```python
from build123d import *

# Parameters (mm, degrees)
BOSS_EXTRUDE1_DEPTH   = 8
CUT_EXTRUDE2_DEPTH    = 27.019223663
M3X0_5_TAPPED_HOLE1_D = 2.5
SKETCH7_W             = 20.825163494
SKETCH7_H             = 21.535112249
CUT_EXTRUDE3_DEPTH    = 8


with BuildPart() as part:
    # Sketch1 → Boss-Extrude1 (new body)
    with BuildSketch(Plane(origin=(0, 0, 0), x_dir=(0, 0, -1), z_dir=(1, 0, 0))):
        Polygon((0, 0), (0, 12), (-17, 18), (-17, 0), align=None)
    boss_extrude1 = extrude(amount=BOSS_EXTRUDE1_DEPTH)

    # Sketch3 → Cut-Extrude2 (cut, through all)
    with BuildSketch(Plane(origin=(0, 0, 0), x_dir=(-1, 0, 0), z_dir=(0, 0, -1))):
        Polygon((-8, 0), (-5, 0), (-3, 4), (-8, 4), align=None)
    cut_extrude2 = extrude(amount=-CUT_EXTRUDE2_DEPTH, mode=Mode.SUBTRACT)

    # M3x0.5 Tapped Hole1 (through all)
    with Locations(Plane(origin=(8, 7, 3), x_dir=(0, 0, 1), z_dir=(1, 0, 0))):
        with Locations((0, 0)):
            m3x0_5_tapped_hole1 = Hole(M3X0_5_TAPPED_HOLE1_D / 2)

    # Mirror1: Boss-Extrude1, Cut-Extrude2, M3x0.5 Tapped Hole1 across plane
    add(boss_extrude1.mirror(Plane(origin=(0, 0, 0), x_dir=(0, 0, 1), z_dir=(1, 0, 0))))
    add(cut_extrude2.mirror(Plane(origin=(0, 0, 0), x_dir=(0, 0, 1), z_dir=(1, 0, 0))), mode=Mode.SUBTRACT)
    add(m3x0_5_tapped_hole1.mirror(Plane(origin=(0, 0, 0), x_dir=(0, 0, 1), z_dir=(1, 0, 0))), mode=Mode.SUBTRACT)

    # Sketch7 → Cut-Extrude3 (cut)
    with BuildSketch(Plane(origin=(8, 0, 0), x_dir=(0, 0, -1), z_dir=(1, 0, 0))):
        with Locations((-8.18446722, 8.52670083)):
            Rectangle(SKETCH7_W, SKETCH7_H)
    extrude(amount=-CUT_EXTRUDE3_DEPTH, mode=Mode.SUBTRACT)


solid = part.part
```
Work out the finished part from the listing and answer in its coordinate system (mm). A direction names the side the tool comes from. Coordinates: 2 decimals unless noted, no trailing zeros. Write each loop counter-clockwise with the first axis right and the second up, starting at its lowest first coordinate (ties: lowest second). Pieces come first, ordered by that corner, then holes. Notation, with made-up numbers: (69, 73) - (81, 73) arc R17 cw to (81, 103) - close; hole circle Ø3 at (25, 51). An arc over 180 degrees is marked (long way). Answer as a JSON object with one key per item and string values.
Q1. Find section A-A (y = 6). Write down the section's boundary in (x, z).
Results list:
{"outline": "(-8, 0) - (0, 0) - (0, 2.25) - (-8, 2.25) - close; (-8, 3.75) - (0, 3.75) - (0, 17) - (-8, 17) - close"}
Q2. Given pin 1 Ø1 at (x, z) = (-6.5, 5.5) entering from -Y; pin 2 Ø1.5 at (y, z) = (7, 3) entering from +X, each flat-ended and moving along its own axis, determine where each tip first touches the part or whether it passes through.
Results list:
{"pin 1": "stops at y = 4", "pin 2": "passes through"}
Q3. Which of the six approach directions +Z, -Z, +X, -X, +Y, -Y give full straight-line access (tool end or side, diameter ignored) to faces 1 (the flat face through (-4, 9, 17)), 2 (the flat face through (-5, 4, 8))?
Results list:
{"face 1": "+Z, +X, -X, +Y, -Y", "face 2": "+Z, -Z, -X"}
Q4. Find section C-C (x = -2). Write down the section's boundary in (y, z).
Results list:
{"outline": "(0, 0) - (12, 0) - (18, 17) - (0, 17) - close; hole circle Ø2.5 at (7, 3)"}
Q5. Consider L1, parallel to Z at x = -2.25, y = 7; L2, parallel to Y at x = -3.25, z = 3; L3, parallel to Y at x = -5.5, z = 3. Determine where each line is inside the solid, lowest interval first. Write a range as from..to.
Results list:
{"L1": "z = 0..1.75, 4.25..17", "L2": "y = 0..3.5, 4..5.75, 8.25..13.06", "L3": "y = 4..5.75, 8.25..13.06"}
Q6. Find section D-D (y = 3). Write down the section's boundary in (x, z).
Results list:
{"outline": "(-3.5, 0) - (0, 0) - (0, 17) - (-3.5, 17) - close"}
Q7. For a pull along Y with two mould halves and no side action, classify faces 3 (the flat face through (-8, 10, 11)), 4 (the cylindrical face through (-4.056, 7.479, 1.845)), 5 (the flat face through (-3.944, 14.958, 8.381)) as pulls with the +Y half, pulls with the -Y half, needs draft (parallel to the pull), parting line crosses it, or undercut.
Results list:
{"face 3": "needs draft", "face 4": "undercut", "face 5": "pulls with the +Y half"}
Q8. Find section B-B (z = 2.75). Write down the section's boundary in (x, y).
Results list:
{"outline": "(-8, 4) - (-3, 4) - (-5, 0) - (0, 0) - (0, 5.78) - (-8, 5.78) - close; (-8, 8.22) - (0, 8.22) - (0, 12.97) - (-8, 12.97) - close"}
